```python
from build123d import *

# Parameters (mm, degrees)
F0_R      = 13
F3_DEPTH  = 7
F2_R      = 19
F4_DEPTH  = 1
F3_FACE_R = 13
F4_FACE_R = 19
F6_T      = -2
F7_R      = 10
F9_R      = 10
F10_R     = 2


# Not quite as in the source:
# - a fillet or chamfer that OpenCascade refuses, or shapes differently, is made with other operations: its cross-section is extruded or revolved along the edge and cut away or added


with BuildPart() as f3:
    # F0 (on Top) → F3 (new body)
    with BuildSketch(Plane.XY):
        Circle(F0_R)
    extrude(amount=F3_DEPTH)



with BuildPart() as f4:
    # F2 (on offset) → F4 (new body)
    with BuildSketch(Plane.XY.offset(15)):
        Circle(F2_R)
    extrude(amount=F4_DEPTH)


with BuildPart() as f3_1:
    add(f3.part)

    add(f4.part)  # F5 merges F4
    # F3_face (on face) → F5 section 0
    with BuildSketch(Plane.XY.offset(7)):
        Circle(F3_FACE_R)
    # F4_face (on face) → F5 section 1
    with BuildSketch(Plane(origin=(0, 0, 15), x_dir=(1, 0, 0), z_dir=(0, 0, -1))):
        Circle(F4_FACE_R)
    loft()

    # F6
    f6_openings = [f3_1.faces().sort_by_distance(p)[0] for p in [
        (0, 0, 16),
        (0, 0, 0),
    ]]
    offset(amount=F6_T, openings=f6_openings, kind=Kind.INTERSECTION)

    # F7
    f7_edges = [f3_1.edges().sort_by_distance(p)[0] for p in [
        (-13, 0, 7),
    ]]
    fillet(f7_edges, radius=F7_R)

    # F8: fillet of radius 5 on 2 edges, made by hand

    # F8_s1 → F8_t2 (revolve, cut)
    with BuildSketch(Plane.XZ):
        with BuildLine():
            ThreePointArc((18.7950549357, 16), (17.8821840065, 15.9159604013), (17, 15.6666666667))
            Line((17, 15.6666666667), (17, 16))
            Line((17, 16), (18.7950549357, 16))
        make_face()
    revolve(axis=Axis((0, 0, 16), (0, 0, -1)), mode=Mode.SUBTRACT)

    # F9
    f9_edges = [f3_1.edges().sort_by_distance(p)[0] for p in [
        (-11, 0, 7.666667),
    ]]
    fillet(f9_edges, radius=F9_R)

    # F10
    f10_edges = [f3_1.edges().sort_by_distance(p)[0] for p in [
        (-17, 0, 15.666667),
    ]]
    fillet(f10_edges, radius=F10_R)


solid = f3_1.part
```
Part model, mm, in its own coordinate system. Round coordinates to 2 decimals unless told otherwise and drop trailing zeros. Order: outer loops, then holes, each group sorted by start corner. A loop starts at its lowest first (then second) coordinate and runs counter-clockwise, first axis right, second up. Notation, with made-up numbers: M 75,-38 L 111,-38 A23 cw 111,-18 Z; hole C 46,89.25 d11. An arc over 180 degrees is marked long. Answer in a Markdown table with one row per item. Add a question column.
Q1. Cut at A-A on z = 13. Give the cut face in (x, y).
Q2. Pin check, flat tips, straight feed: pin 1 (8 mm diameter, centred on x = 9.5, z = 2, fed in from +Y); pin 2 (4 mm diameter, centred on y = 9, z = 10.5, fed in from -X); pin 3 (4 mm diameter, centred on y = -2.5, z = 12, fed in from -X). Stop position of each tip, or through.
Q3. Wall check: L1, parallel to Y at x = 0, z = 1.8; L2, parallel to Y at x = 2, z = 3.75. Give the ranges that are in metal, low to high. Write a range as from..to.
Q4. Mould opens along Y. For faces 1 (the face through (-11, 3, 0)), 2 (the face through (-2.82, -12.69, 1.81)), 3 (the face through (-2.38, -10.74, 2.14)) say: +Y half, -Y half, draft (parallel to the pull), parting line (faces both ways), or undercut.
Established:
| question | item | result |
|---|---|---|
| 1 | outline | C 0,0 d35; hole C 0,0 d30 |
| 2 | pin 1 | stops at y = 11.78 |
| 2 | pin 2 | stops at x = -14.92 |
| 2 | pin 3 | stops at x = -18.1 |
| 3 | L1 | y = -13..-11, 11..13 |
| 3 | L2 | y = -12.85..-10.82, 10.82..12.85 |
| 4 | face 1 | draft |
| 4 | face 2 | parting line |
| 4 | face 3 | undercut |
